Geometry check sheet. Reference: the model listing, model coordinates, mm. A direction names the side the tool comes from. Give positions to 0.01 mm unless a question says otherwise; leave off trailing zeros. Loops run counter-clockwise (first coordinate to the right, second up) from the corner with the lowest first, then second, coordinate; pieces in that order, holes last. Notation, with made-up numbers: (3.25, 35.25) -> (33.25, 35.25) arc R32 ccw to (33.25, 61.25) -> close; hole circle Ø5 at (81, 25.25). An arc over 180 degrees is marked (long way). Answer as a JSON object with one key per item and string values.
from build123d import *

# Parameters (mm, degrees)
SKETCH1_W           = 44.45
SKETCH1_H           = 50.8
SKETCH1_R           = 6.5
SKETCH1_R_2         = 1.5
BOSS_EXTRUDE1_DEPTH = 3.175
SKETCH2_W           = 44.45
SKETCH2_H           = 3.175
BOSS_EXTRUDE2_DEPTH = 47.625
SKETCH3_R           = 3.175
CUT_EXTRUDE1_DEPTH  = 4.175


with BuildPart() as part:
    # Sketch1 → Boss-Extrude1 (new body)
    with BuildSketch(Plane.XY):
        with Locations((22.225, 25.4)):
            Rectangle(SKETCH1_W, SKETCH1_H)
        with Locations((22.225, 32.4)):
            Circle(SKETCH1_R, mode=Mode.SUBTRACT)
        with Locations((6.725, 25.4)):
            Circle(SKETCH1_R_2, mode=Mode.SUBTRACT)
        with Locations((37.725, 25.4)):
            Circle(SKETCH1_R_2, mode=Mode.SUBTRACT)
        with Locations((29.975, 11.976606241)):
            Circle(SKETCH1_R_2, mode=Mode.SUBTRACT)
        with Locations((14.475, 11.976606241)):
            Circle(SKETCH1_R_2, mode=Mode.SUBTRACT)
        with Locations((14.475, 38.823393759)):
            Circle(SKETCH1_R_2, mode=Mode.SUBTRACT)
        with Locations((29.975, 38.823393759)):
            Circle(SKETCH1_R_2, mode=Mode.SUBTRACT)
    extrude(amount=BOSS_EXTRUDE1_DEPTH)

    # Sketch2 → Boss-Extrude2 (add)
    with BuildSketch(Plane(origin=(0, 0, 0), x_dir=(-1, 0, 0), z_dir=(0, 0, -1))):
        with Locations((-22.225, 1.5875)):
            Rectangle(SKETCH2_W, SKETCH2_H)
    extrude(amount=BOSS_EXTRUDE2_DEPTH)

    # Sketch3 → Cut-Extrude1 (cut, through all)
    with BuildSketch(Plane(origin=(0, 3.175, 0), x_dir=(1, 0, 0), z_dir=(0, 1, 0))):
        with Locations((34.925, 9.525)):
            Circle(SKETCH3_R)
        with Locations((34.925, 34.925)):
            Circle(SKETCH3_R)
        with Locations((9.525, 9.525)):
            Circle(SKETCH3_R)
        with Locations((9.525, 34.925)):
            Circle(SKETCH3_R)
    extrude(amount=-CUT_EXTRUDE1_DEPTH, mode=Mode.SUBTRACT)


solid = part.part
1) Tool access check on faces 5 (the face through (23, 3.175, -23)), 6 (the face through (36.632, 1.61, -37.602)). Record the directions out of +Z, -Z, +X, -X, +Y, -Y that give a thin tool (end or side, any length) a straight path to the whole face; none if there is none.
Geometry check:
{"face 5": "-Z, +X, -X, +Y", "face 6": "+Y, -Y"}
2) Depth check by flat-ended pin: P1, Ø6, axis at x = 37.5, z = -15, coming from the +Y side (3 decimals); P2, Ø3.5, axis at x = 37.725, y = 25.4, coming from the -Z side. Enter the tip coordinate at first touch or a pass-through.
Geometry check:
{"P1": "stops at y = 3.175", "P2": "stops at z = 0"}
3) Material ranges on line 1 along Z through (x, y) = (36.5, 21.5) (3 decimals), recorded low to high. Write a range as from..to.
Geometry check:
{"line 1": "z = 0..3.175"}
4) Draft check along Z on faces 1 (the face through (11.232, 1.61, -12.202)), 2 (the face through (11.232, 1.61, -37.602)), 3 (the face through (21.914, 25.756, 3.175)), 4 (the face through (22, 50.8, 2)). Enter one of: pulls with the +Z half, pulls with the -Z half, needs draft (parallel to the pull), parting line crosses it, or undercut.
Geometry check:
{"face 1": "undercut", "face 2": "undercut", "face 3": "pulls with the +Z half", "face 4": "needs draft"}
5) Section check B-B on x = 11. Record the cut outline in (y, z) (3 decimals), plus the area to 3 significant figures.
Geometry check:
{"outline": "(0, -47.625) -> (3.175, -47.625) -> (3.175, -37.737) -> (0, -37.737) -> close; (0, -32.113) -> (3.175, -32.113) -> (3.175, -12.337) -> (0, -12.337) -> close; (0, -6.713) -> (3.175, -6.713) -> (3.175, 0) -> (50.8, 0) -> (50.8, 3.175) -> (0, 3.175) -> close", "area": "277 mm2"}
6) Section check A-A on y = 32.4. Record the cut outline in (x, z) (3 decimals).
Geometry check:
{"outline": "(0, 0) -> (15.725, 0) -> (15.725, 3.175) -> (0, 3.175) -> close; (28.725, 0) -> (44.45, 0) -> (44.45, 3.175) -> (28.725, 3.175) -> close"}
7) Section check C-C on y = 7. Record the cut outline in (x, z) (3 decimals), plus the area to 3 significant figures.
Geometry check:
{"outline": "(0, 0) -> (44.45, 0) -> (44.45, 3.175) -> (0, 3.175) -> close", "area": "141 mm2"}
